```python
from build123d import *

# Parameters (mm, degrees)
BOSS_EXTRUDE1_DEPTH = 3.35
SKETCH2_R           = 2
CUT_EXTRUDE1_DEPTH  = 6.7


with BuildPart() as part:
    # Sketch1 → Boss-Extrude1 (new body, symmetric)
    with BuildSketch(Plane(origin=(0, 0, 0), x_dir=(0, 0, -1), z_dir=(1, 0, 0))):
        with BuildLine():
            ThreePointArc((0, 0), (10.830584713, -1.585060066), (20.752730266, -6.207289856))
            ThreePointArc((20.752730266, -6.207289856), (24.907289856, -5.347269734), (24.047269734, -1.192710144))
            ThreePointArc((24.047269734, -1.192710144), (12.549962758, 4.163308324), (0, 6))
            ThreePointArc((0, 6), (-12.549962758, 4.163308324), (-24.047269734, -1.192710144))
            ThreePointArc((-24.047269734, -1.192710144), (-24.907289856, -5.347269734), (-20.752730266, -6.207289856))
            ThreePointArc((-20.752730266, -6.207289856), (-10.830584713, -1.585060066), (0, 0))
        make_face()
    extrude(amount=BOSS_EXTRUDE1_DEPTH, both=True)

    # Sketch2 → Cut-Extrude1 (cut)
    with BuildSketch(Plane(origin=(3.35, 0, 0), x_dir=(0, 0, -1), z_dir=(1, 0, 0))):
        with Locations((-22.4, -3.7)):
            Circle(SKETCH2_R)
        with Locations((22.4, -3.7)):
            Circle(SKETCH2_R)
    extrude(amount=-CUT_EXTRUDE1_DEPTH, mode=Mode.SUBTRACT)


solid = part.part
```
The listing builds one solid part. Answer for the finished solid, in the listing's coordinates (mm). Round coordinates to 2 decimals unless told otherwise and drop trailing zeros. Order: outer loops, then holes, each group sorted by start corner. A loop starts at its lowest first (then second) coordinate and runs counter-clockwise, first axis right, second up. Notation, with made-up numbers: (-22, 88) - (6, 88) arc R4 ccw to (6, 93) - close; hole circle Ø3 at (79, -28). An arc over 180 degrees is marked (long way). Put each result on its own line as item: value. Start each with the question number.
(1) Find section A-A (y = -4.25). Give the vertices of the cut face in (x, z).
(2) Find section B-B (z = 22.4). Give the vertices of the cut face in (x, y).
(3) Straight lines are drawn through the part: probe 1 along Y at (x, z) = (0, 22.4); probe 2 along Z at (x, y) = (1.25, 1); probe 3 along Z at (x, y) = (1.5, 1.75). For each, find the intervals that lie inside material, in ascending order. Write a range as from..to.
(4) Determine the mould class of faces 1 (the flat face through (3.35, 1, 0)), 2 (the cylindrical face through (0.047, -3.099, 20.492)), 3 (the cylindrical face through (0.05, -5.4, -24.87)), 4 (the cylindrical face through (0, 6, 0)) for opening direction Z: released by +Z, released by -Z, zero draft, split by the parting line, or undercut.
(5) Find section D-D (z = 14). Give the vertices of the cut face in (x, y).
(6) Given P1, Ø4, axis at x = -1.5, z = -7.5, coming from the -Y side; P2, Ø4, axis at y = -4.5, z = -12, coming from the -X side, each flat-ended and moving along its own axis, determine where each tip first touches the part or whether it passes through.
(7) Find section C-C (x = -2.5). Give the vertices of the cut face in (y, z).
Reply:
1. outline: (-3.35, -25.35) - (3.35, -25.35) - (3.35, -24.32) - (-3.35, -24.32) - close; (-3.35, -20.48) - (3.35, -20.48) - (3.35, -17.41) - (-3.35, -17.41) - close; (-3.35, 17.41) - (3.35, 17.41) - (3.35, 20.48) - (-3.35, 20.48) - close; (-3.35, 24.32) - (3.35, 24.32) - (3.35, 25.35) - (-3.35, 25.35) - close
2. outline: (-3.35, -6.7) - (3.35, -6.7) - (3.35, -5.7) - (-3.35, -5.7) - close; (-3.35, -1.7) - (3.35, -1.7) - (3.35, -0.16) - (-3.35, -0.16) - close
3. probe 1: -6.7..-5.7, -1.7..-0.16
3. probe 2: -20.32..20.32
3. probe 3: -18.82..18.82
4. face 1: zero draft
4. face 2: undercut
4. face 3: undercut
4. face 4: split by the parting line
5. outline: (-3.35, -2.69) - (3.35, -2.69) - (3.35, 3.7) - (-3.35, 3.7) - close
6. P1: y = -1.21
6. P2: through
7. outline: (-6.21, -20.75) arc R3 ccw to (-1.19, -24.05) arc R43.79 ccw to (-1.19, 24.05) arc R3 ccw to (-6.21, 20.75) arc R37.79 cw to start; hole circle Ø4 at (-3.7, -22.4); hole circle Ø4 at (-3.7, 22.4)
